Source: CAD feature listing. Evaluate the final solid. Frame: model axes, mm. Coordinates: 2 decimals unless noted, no trailing zeros. Order: outer loops, then holes, each group sorted by start corner. A loop starts at its lowest first (then second) coordinate and runs counter-clockwise, first axis right, second up.
```python
from build123d import *

# Parameters (mm, degrees)
SKETCH1_R           = 2.5
BOSS_EXTRUDE1_DEPTH = 4


with BuildPart() as part:
    # Sketch1 → Boss-Extrude1 (new body)
    with BuildSketch(Plane.XY):
        Polygon((181.321497127, 204.5460303), (-226.678502873, 204.5460303), (-226.678502873, -253.4539697), (181.321497127, -253.4539697), (181.321497127, -145.4539697), (131.321497127, -145.4539697), (131.321497127, 96.5460303), (181.321497127, 96.5460303), align=None)
        with Locations((-214.178502873, -215.246862919)):
            Circle(SKETCH1_R, mode=Mode.SUBTRACT)
        with Locations((-188.471396092, -240.907728533)):
            Circle(SKETCH1_R, mode=Mode.SUBTRACT)
        with Locations((-22.324949482, -240.60041631)):
            Circle(SKETCH1_R, mode=Mode.SUBTRACT)
        with Locations((143.821776426, -240.640809696)):
            Circle(SKETCH1_R, mode=Mode.SUBTRACT)
        with Locations((168.874598055, -215.554555333)):
            Circle(SKETCH1_R, mode=Mode.SUBTRACT)
        with Locations((169.487625208, 166.030738683)):
            Circle(SKETCH1_R, mode=Mode.SUBTRACT)
        with Locations((143.821776426, 191.732870295)):
            Circle(SKETCH1_R, mode=Mode.SUBTRACT)
        with Locations((-22.324949482, 191.692476909)):
            Circle(SKETCH1_R, mode=Mode.SUBTRACT)
        with Locations((-188.471396092, 191.999789133)):
            Circle(SKETCH1_R, mode=Mode.SUBTRACT)
        with Locations((-214.178502873, 166.338923519)):
            Circle(SKETCH1_R, mode=Mode.SUBTRACT)
        with Locations((-214.178502873, -24.4539697)):
            Circle(SKETCH1_R, mode=Mode.SUBTRACT)
    extrude(amount=BOSS_EXTRUDE1_DEPTH)


solid = part.part
```
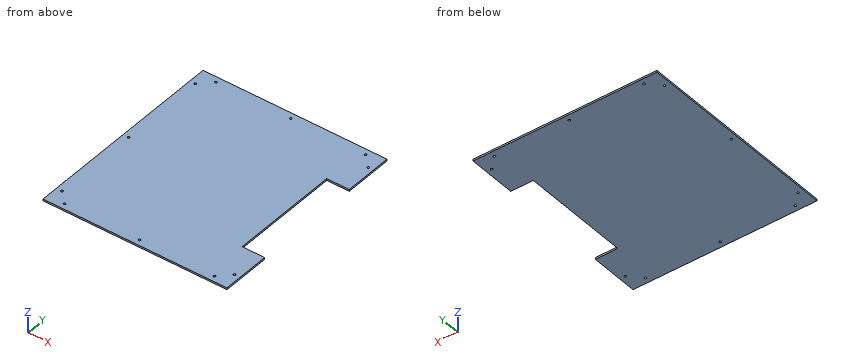
Q1. Section query B-B on y = -97.5. Output: boundary loops of the cut face in (x, z), plus the area to 3 significant figures.
Solutions:
outline: (-226.68, 0) - (131.32, 0) - (131.32, 4) - (-226.68, 4) - close
area: 1,430 mm2
Q2. Material intervals for line 1 along X through (y, z) = (60, 3.45); line 2 along Y through (x, z) = (145, 3.4), sorted ascending.
Solutions:
line 1: x = -226.68 to 131.32
line 2: y = -253.45 to -242.85, -238.44 to -145.45, 96.55 to 189.53, 193.94 to 204.55
Q3. Section query A-A on z = 1.45. Give the number of separate pieces and of enclosed holes in the cut face, plus the area to 3 significant figures.
Solutions:
separate pieces: 1
enclosed holes: 11
area: 175,000 mm2
Q4. Pin query (flat end, axial travel): P1, Ø1.5, axis at y = -5.5, z = 2, coming from the +X side. Return the tip coordinate at first contact, or that it passes through.
Solutions:
P1: stops at x = 131.32
